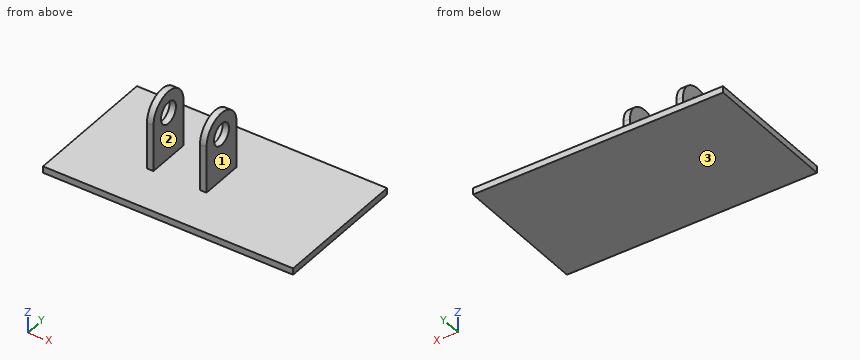
Autodesk Inventor part; units mm, degrees
ref_plane "YZ Plane" through (0, 0, 0) normal (1, 0, 0) x (0, 1, 0)
ref_plane "XZ Plane" through (0, 0, 0) normal (0, 1, 0) x (-1, 0, 0)
ref_plane "XY Plane" through (0, 0, 0) normal (0, 0, 1) x (1, 0, 0)
sketch "Sketch2" plane through (0, 0, 0) normal (1, 0, 0) x (0, 1, 0)
  line L0 (20, 27.3876) -> (-42.6897, 27.3876)
  line L1 (-42.6897, 21.3876) -> (20, 21.3876)
  line L2 (20, 21.3876) -> (20, 27.3876)
  line L3 (-42.6897, -21.3876) -> (20, -21.3876)
  line L4 (20, -21.3876) -> (20, -27.3876)
  line L5 (20, -27.3876) -> (-42.6897, -27.3876)
  line L6 (-42.6897, -93.6124) -> (-48.6897, -93.6124)
  line L7 (-48.6897, -93.6124) -> (-48.6897, 136.3876)
  line L8 (-48.6897, 136.3876) -> (-42.6897, 136.3876)
  line L9 (-42.6897, 136.3876) -> (-42.6897, 27.3876)
  line L10 (-42.6897, 21.3876) -> (-42.6897, -21.3876)
  line L11 (-42.6897, -27.3876) -> (-42.6897, -93.6124)
  point P0 (0, 0)
  dimension "d3" = 6
  dimension "d5" = 48.6897
  dimension "d6" = 136.3876
  dimension "d7" = 93.6124
  dimension "d9" = 27.3876
  dimension "d10" = 27.3876
  dimension "d11" = 20
extrude "Extrusion1" add sketch "Sketch2" along normal mid plane 125
sketch "Sketch3" plane through (-62.5, -42.6897, 27.3876) normal (0, 0, 1) x (1, 0, 0)
  circle A0 centre (62.5, 42.6897) radius 10
  dimension "d14" = 20
extrude "Extrusion2" cut sketch "Sketch3" against normal through all
sketch "Sketch4" plane through (-62.5, -42.6897, 27.3876) normal (0, 0, 1) x (1, 0, 0)
  circle A0 centre (62.5, 42.6897) radius 10
  line L0 (0, 0) -> (125, 0)
  line L1 (125, 62.6897) -> (125, 0)
  line L2 (125, 62.6897) -> (0, 62.6897)
  line L3 (0, 0) -> (0, 62.6897)
  arc A1 (82.5, 42.6897) -> (42.5, 42.6897) centre (62.5, 42.6897) ccw
  line L4 (42.5, 42.6897) -> (42.5, 0)
  line L5 (82.5, 0) -> (82.5, 42.6897)
extrude "Extrusion3" cut sketch "Sketch4" against normal through all contours L3 L2 A1 L4 L0 | L5 A1 L2 L1 L0
move or copy body "Move Body1" bodies to move or copy 1 copy no rotation origin (0, 0, 0) rotation axis (1, 0, 0) rotation angle 90
move or copy body "Move Body2" bodies to move or copy 1 copy no rotation origin (0, 0, 0) rotation axis (0, 0, 1) rotation angle 90
properties part number "Foot"
Geometry check sheet. Reference: the model listing, model coordinates, mm. Face numbers are marked on the shaded views. Coordinates: 2 decimals unless noted, no trailing zeros. Order: outer loops, then holes, each group sorted by start corner. A loop starts at its lowest first (then second) coordinate and runs counter-clockwise, first axis right, second up.
Item 1: Section check D-D (y = 14). Enter the section's corners in (x, z), plus the area to 3 significant figures.
Item 2: Depth check by flat-ended pin: pin 1 (5 mm diameter, centred on x = 23.5, z = -22.5, fed in from +Y); pin 2 (6.5 mm diameter, centred on x = 24.5, z = -29, fed in from -Y); pin 3 (23 mm diameter, centred on y = 0, z = 0, fed in from +X). Enter the tip coordinate at first touch or a pass-through.
Item 3: Mould release check, pull along X, two halves, no side actions. Record for the marked faces 1, 2 and 3: released by +X, released by -X, zero draft, split by the parting line, or undercut.
Item 4: Scan lines: line 1 along X through (y, z) = (15, -35); line 2 along Z through (x, y) = (24.8, 0); line 3 along Z through (x, y) = (7.5, -51). Record each from-to range of solid material in increasing order.
Item 5: Section check C-C (x = -46.5). Enter the section's corners in (y, z).
Item 6: Section check B-B (z = -20). Enter the section's corners in (x, y), plus the area to 3 significant figures.
Item 7: Section check A-A (y = 0). Enter the section's corners in (x, z).
Check sheet entries:
1. outline: (-93.61, -48.69) - (136.39, -48.69) - (136.39, -42.69) - (27.39, -42.69) - (27.39, 14.28) - (21.39, 14.28) - (21.39, -42.69) - (-21.39, -42.69) - (-21.39, 14.28) - (-27.39, 14.28) - (-27.39, -42.69) - (-93.61, -42.69) - close
1. area: 2,060 mm2
2. pin 1: stops at y = 20
2. pin 2: stops at y = -20
2. pin 3: stops at x = 27.39
3. face 1: released by +X
3. face 2: undercut
3. face 3: zero draft
4. line 1: x = -27.39 to -21.39, 21.39 to 27.39
4. line 2: z = -48.69 to -10, 10 to 20
4. line 3: z = -48.69 to -42.69
5. outline: (-62.5, -48.69) - (62.5, -48.69) - (62.5, -42.69) - (-62.5, -42.69) - close
6. outline: (-27.39, -20) - (-21.39, -20) - (-21.39, 20) - (-27.39, 20) - close; (21.39, -20) - (27.39, -20) - (27.39, 20) - (21.39, 20) - close
6. area: 480 mm2
7. outline: (-93.61, -48.69) - (136.39, -48.69) - (136.39, -42.69) - (27.39, -42.69) - (27.39, -10) - (21.39, -10) - (21.39, -42.69) - (-21.39, -42.69) - (-21.39, -10) - (-27.39, -10) - (-27.39, -42.69) - (-93.61, -42.69) - close; (-27.39, 10) - (-21.39, 10) - (-21.39, 20) - (-27.39, 20) - close; (21.39, 10) - (27.39, 10) - (27.39, 20) - (21.39, 20) - close
